```python
from build123d import *

# Parameters (mm, degrees)
SKETCH1_W           = 19.05
SKETCH1_H           = 76.2
REVOLVE1_ANGLE      = 180
SKETCH2_W           = 38.1
SKETCH2_H           = 76.2
BOSS_EXTRUDE1_DEPTH = 330.2
SKETCH3_R           = 3.9878
CUT_EXTRUDE1_DEPTH  = 342.013328185


with BuildPart() as part:
    # Sketch1 → Revolve1 (revolve)
    with BuildSketch(Plane.XY):
        with Locations((9.525, -38.1)):
            Rectangle(SKETCH1_W, SKETCH1_H)
    revolve(axis=Axis((19.05, 0, 0), (0, -1, 0)), revolution_arc=REVOLVE1_ANGLE)

    # Sketch2 → Boss-Extrude1 (add)
    with BuildSketch(Plane.XY):
        with Locations((19.05, -38.1)):
            Rectangle(SKETCH2_W, SKETCH2_H)
    extrude(amount=BOSS_EXTRUDE1_DEPTH)

    # Sketch3 → Cut-Extrude1 (cut, through all)
    with BuildSketch(Plane(origin=(0, 0, 0), x_dir=(1, 0, 0), z_dir=(0, 1, 0))):
        with Locations(Location((19.05, 0, 0), (0, 0, 180))):
            Circle(SKETCH3_R)
    extrude(amount=-CUT_EXTRUDE1_DEPTH, mode=Mode.SUBTRACT)


solid = part.part
```
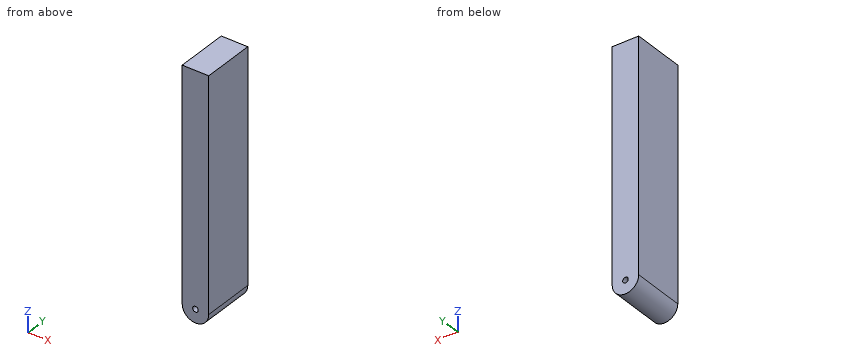
Can you work these out from the model? Positions are in its coordinate system, mm. Coordinates: 2 decimals unless noted, no trailing zeros. Write each loop counter-clockwise with the first axis right and the second up, starting at its lowest first coordinate (ties: lowest second). Pieces come first, ordered by that corner, then holes. Notation, with made-up numbers: (4, 60.25) - (31, 60.25) arc R11 cw to (31, 71.25) - close; hole circle Ø8 at (37.25, 88.5). An arc over 180 degrees is marked (long way). Return JSON: item names as keys, results as strings.
Q1. If we section it at B-B (y = -10.5): Please give me the cut outline in (x, z).
Computed values:
{"outline": "(0, 0) arc R19.05 ccw to (38.1, 0) - (38.1, 330.2) - (0, 330.2) - close; hole circle Ø7.98 at (19.05, 0)"}
Q2. I'm going to push flat-ended pins straight in: pin 1 Ø1 at (x, y) = (26, -40) entering from -Z; pin 2 Ø12 at (x, y) = (25, -7.5) entering from -Z; pin 3 Ø7 at (x, z) = (19.05, 0) entering from +Y. Where does each tip first touch, or does it pass through?
Computed values:
{"pin 1": "stops at z = -17.92", "pin 2": "stops at z = -19.05", "pin 3": "passes through"}
Q3. If we section it at A-A (x = 19.05): Please give me the cut outline in (y, z).
Computed values:
{"outline": "(-76.2, -19.05) - (0, -19.05) - (0, -3.99) - (-76.2, -3.99) - close; (-76.2, 3.99) - (0, 3.99) - (0, 330.2) - (-76.2, 330.2) - close"}
Q4. Please list where these lines run through material, in increasing order: L1, parallel to Z at x = 19.05, y = -36.5; L2, parallel to Z at x = 21, y = -25.5; L3, parallel to Z at x = 6, y = -13.5. Write a range as from..to.
Computed values:
{"L1": "z = -19.05..-3.99, 3.99..330.2", "L2": "z = -18.95..-3.48, 3.48..330.2", "L3": "z = -13.88..330.2"}
